Here's how the part is built. I have some questions about the finished solid (model axes, mm). A direction names the side the tool comes from. Give positions to 0.01 mm unless a question says otherwise; leave off trailing zeros. Loops run counter-clockwise (first coordinate to the right, second up) from the corner with the lowest first, then second, coordinate; pieces in that order, holes last.
Q1. I need wall thicknesses on line 1 (Y direction, x = -17, z = 9.5); line 2 (X direction, y = 4.5, z = -36); line 3 (Z direction, x = -20.5, y = 5.25). Which ranges of each line are inside material? Lowest first, please.
Q2. If we section it at C-C (y = 7): Please give me the cut outline in (x, z), plus the area to 3 significant figures.
Q3. We'd pull the mould along X, two halves only. Please class faces 1 (the face through (27.791, 10.93, 15.864)), 2 (the face through (29.5, 16, 16.8)), 3 (the face through (-12.33, 10.93, -33.88)): +X half, -X half, draft (parallel to the pull), parting line (faces both ways), or undercut.
Q4. For faces 4 (the face through (14.1, 3.04, -8.63)), 5 (the face through (0, 11, -32)), 6 (the face through (0, 6, 2)), which set-ups out of +Z, -Z, +X, -X, +Y, -Y let a thin tool reach every point of the face, with its end or its side?
Q5. If we section it at D-D (z = 14): Please give me the cut outline in (x, y), plus the area to 3 significant figures.
Q6. If we section it at B-B (z = 23.5): Please give me the cut outline in (x, y), plus the area to 3 significant figures.
Q7. If we section it at A-A (x = 0): Please give me the cut outline in (y, z).
Q8. Will these pins go through, and if not, where does the flat tip stop? P1, Ø5, axis at x = 1, y = 12, coming from the +Z side; P2, Ø3, axis at x = 21, y = 4.5, coming from the -Z side; P3, Ø3, axis at x = 30, y = 12, coming from the +Z side.
from build123d import *

# Parameters (mm, degrees)
SKETCH1_R           = 40
BOSS_EXTRUDE1_DEPTH = 6
SKETCH2_R           = 1.5
BOSS_EXTRUDE2_DEPTH = 10
SKETCH16_R          = 1.5
CUT_EXTRUDE9_DEPTH  = 17
CIRPATTERN1_COUNT   = 3
SKETCH5_R           = 30.471270003
CUT_EXTRUDE3_DEPTH  = 7
CIRPATTERN2_COUNT   = 3


with BuildPart() as part:
    # Sketch1 → Boss-Extrude1 (new body)
    with BuildSketch(Plane(origin=(0, 0, 0), x_dir=(1, 0, 0), z_dir=(0, 1, 0))):
        Circle(SKETCH1_R)
    extrude(amount=BOSS_EXTRUDE1_DEPTH)

    # Sketch2 → Boss-Extrude2 (add)
    with BuildSketch(Plane(origin=(0, 6, 0), x_dir=(1, 0, 0), z_dir=(0, 1, 0))):
        with BuildLine():
            Line((-13.680805733, 37.587704831), (-10.944644586, 30.070163865))
            ThreePointArc((-10.944644586, 30.070163865), (0, 32), (10.944644586, 30.070163865))
            Line((10.944644586, 30.070163865), (13.680805733, 37.587704831))
            ThreePointArc((13.680805733, 37.587704831), (0, 40), (-13.680805733, 37.587704831))
        make_face()
        with Locations((0, 36)):
            Circle(SKETCH2_R, mode=Mode.SUBTRACT)
    boss_extrude2 = extrude(amount=BOSS_EXTRUDE2_DEPTH)

    # Sketch16 → Cut-Extrude9 (cut, through all)
    with BuildSketch(Plane(origin=(0, 16, 0), x_dir=(1, 0, 0), z_dir=(0, 1, 0))):
        with Locations((0, 36)):
            Circle(SKETCH16_R)
    cut_extrude9 = extrude(amount=-CUT_EXTRUDE9_DEPTH, mode=Mode.SUBTRACT)

    # CirPattern1: Boss-Extrude2, Cut-Extrude9 ×3 about axis
    cirpattern1_axis = Axis((0, 0, 0), (0, 1, 0))
    for i in range(1, CIRPATTERN1_COUNT):
        add(boss_extrude2.rotate(cirpattern1_axis, i * 360 / CIRPATTERN1_COUNT))
        add(cut_extrude9.rotate(cirpattern1_axis, i * 360 / CIRPATTERN1_COUNT), mode=Mode.SUBTRACT)

    # Sketch5 → Cut-Extrude3 (cut, through all)
    with BuildSketch(Plane(origin=(0, 6, 0), x_dir=(1, 0, 0), z_dir=(0, 1, 0))):
        with Locations((40.698571494, 23.497331208)):
            Circle(SKETCH5_R)
    cut_extrude3 = extrude(amount=-CUT_EXTRUDE3_DEPTH, mode=Mode.SUBTRACT)

    # CirPattern2: Cut-Extrude3 ×3 about axis
    cirpattern2_axis = Axis((0, 0, 0), (0, 1, 0))
    for i in range(1, CIRPATTERN2_COUNT):
        add(cut_extrude3.rotate(cirpattern2_axis, i * 360 / CIRPATTERN2_COUNT), mode=Mode.SUBTRACT)


solid = part.part
Check sheet entries:
1. line 1: y = 0 to 6
1. line 2: x = -12.91 to -1.5, 1.5 to 12.91
1. line 3: z = -0.68 to 24.45
2. outline: (-39.39, 6.95) - (-31.51, 5.56) arc R32 cw to (-20.57, 24.51) - (-25.71, 30.64) arc R40 ccw to start; (-13.68, -37.59) arc R40 ccw to (13.68, -37.59) - (10.94, -30.07) arc R32 cw to (-10.94, -30.07) - close; (20.57, 24.51) arc R32 cw to (31.51, 5.56) - (39.39, 6.95) arc R40 ccw to (25.71, 30.64) - close; hole circle Ø3 at (-31.18, 18); hole circle Ø3 at (0, -36); hole circle Ø3 at (31.18, 18)
2. area: 582 mm2
3. face 1: undercut
3. face 2: draft
3. face 3: -X half
4. face 4: +X, -Y
4. face 5: +Z, +Y
4. face 6: +Y
5. outline: (-37.47, 0) - (37.47, 0) - (37.47, 16) - (28.77, 16) - (28.77, 6) - (-28.77, 6) - (-28.77, 16) - (-37.47, 16) - close
5. area: 624 mm2
6. outline: (-32.37, 0) - (-19.4, 0) - (-19.4, 6) - (-21.72, 6) - (-21.72, 16) - (-32.37, 16) - close; (19.4, 0) - (32.37, 0) - (32.37, 16) - (21.72, 16) - (21.72, 6) - (19.4, 6) - close
6. area: 369 mm2
7. outline: (0, -40) - (16, -40) - (16, -37.5) - (0, -37.5) - close; (0, -34.5) - (16, -34.5) - (16, -32) - (6, -32) - (6, 16.52) - (0, 16.52) - close
8. P1: stops at z = -31.81
8. P2: stops at z = -1.61
8. P3: stops at z = 28.07
